Part model, mm, in its own coordinate system. Round coordinates to 2 decimals unless told otherwise and drop trailing zeros. Write each loop counter-clockwise with the first axis right and the second up, starting at its lowest first coordinate (ties: lowest second). Pieces come first, ordered by that corner, then holes.
from build123d import *

# Parameters (mm, degrees)
SKETCH2_R          = 4
CUT_EXTRUDE1_DEPTH = 10


with BuildPart() as part:
    # Sketch1 → Revolve1 (revolve)
    with BuildSketch(Plane(origin=(0, 0, 0), x_dir=(1, 0, 0), z_dir=(0, 1, 0)), mode=Mode.PRIVATE) as revolve1_sk:
        Polygon((5, 0), (-5, 0), (-5, 25), (-2.5, 25), (0, 15), (2.5, 25), (5, 25), align=None)
    revolve(revolve1_sk.sketch.rotate(Axis((-18.958333333, 0, 0), (1, 0, 0)), 180), axis=Axis((-18.958333333, 0, 0), (1, 0, 0)))

    # Sketch2 → Cut-Extrude1 (cut)
    with BuildSketch(Plane.ZY.offset(5)):
        Circle(SKETCH2_R)
    extrude(amount=-CUT_EXTRUDE1_DEPTH, mode=Mode.SUBTRACT)


solid = part.part
Q1. Wall check: line 1 (X direction, y = -13.5, z = -21); line 2 (X direction, y = 19, z = -1); line 3 (Z direction, x = 4.25, y = -22). Give the ranges that are in metal, low to high.
Q2. Drop flat-ended pins along their axis: P1, Ø5, axis at x = -2, z = 12.5, coming from the +Y side; P2, Ø1, axis at x = -3, y = -4.5, coming from the -Z side; P3, Ø6, axis at x = 2.5, z = 3, coming from the +Y side. Give the stop position or say it passes through.
Q3. Two-plate mould, pull along X, no slides. Class faces 1 (the conical face through (-0.12, -4.65, 14.77)), 2 (the flat face through (-5, 5, 0)), 3 (the conical face through (0.156, 13.863, 7.21)), 4 (the flat face through (5, 5, 0)): released by +X, released by -X, zero draft, split by the parting line, or undercut.
Q4. Saw through at D-D, the plane x = -1.5. Write the cut outline in (y, z).
Q5. Saw through at C-C, the plane x = 1.75. Write the cut outline in (y, z).
Q6. Saw through at A-A, the plane y = 0. Write the cut outline in (x, z), and give its area (3 significant figures).
Computed:
1. line 1: x = -5 to -2.49, 2.49 to 5
1. line 2: x = -5 to -1.01, 1.01 to 5
1. line 3: z = -11.87 to 11.87
2. P1: stops at y = 22.89
2. P2: stops at z = -24.68
2. P3: stops at y = 25
3. face 1: undercut
3. face 2: released by -X
3. face 3: undercut
3. face 4: released by +X
4. outline: circle Ø42 at (0, 0); hole circle Ø8 at (0, 0)
5. outline: circle Ø44 at (0, 0); hole circle Ø8 at (0, 0)
6. outline: (-5, -25) - (-2.5, -25) - (0, -15) - (2.5, -25) - (5, -25) - (5, -4) - (-5, -4) - close; (-5, 4) - (5, 4) - (5, 25) - (2.5, 25) - (0, 15) - (-2.5, 25) - (-5, 25) - close
6. area: 370 mm2
